For this review, take the finished solid that the model builds, in its own axes (mm). Face numbers are marked on the shaded views. Round coordinates to 2 decimals unless told otherwise and drop trailing zeros. Loops run counter-clockwise (first coordinate to the right, second up) from the corner with the lowest first, then second, coordinate; pieces in that order, holes last.
1) Mouldability with a two-part tool opening along X and no side actions: class the marked faces 1, 2 and 3 as pulls with the +X half, pulls with the -X half, needs draft (parallel to the pull), parting line crosses it, or undercut.
2) Insertion check: pin 1 (3 mm diameter, centred on x = 44.45, y = 780.22, fed in from -Z). The pin has a flat end and moves straight along its axis. Give the tip position at first contact, or say it passes through.
3) Take a section at A-A (z = 134.75). State the section outline as (x, y) points.
4) Take a section at B-B (x = 44). Give the number of separate pieces and of enclosed holes in the cut face, then the cut area to 3 significant figures.
5) Wall thickness on L1, parallel to Y at x = 41, z = 135; L2, parallel to Y at x = 40.25, z = 134.5; L3, parallel to Y at x = 46, z = 136: over which ranges is each line inside the solid? List them lowest first.
6) Take a section at C-C (z = 131.25). State the section outline as (x, y) points.
```python
from build123d import *

# Parameters (mm, degrees)
SKETCH1_W           = 9.525
SKETCH1_H           = 50.8
SKETCH1_R           = 3.175
BOSS_EXTRUDE1_DEPTH = 12.7
CUT_EXTRUDE1_REACH  = 791.849
SKETCH2_R           = 2.6035


with BuildPart() as part:
    # Sketch1 → Boss-Extrude1 (new body)
    with BuildSketch(Plane(origin=(38.1, 0, 0), x_dir=(0, 0, -1), z_dir=(1, 0, 0))):
        with Locations((-134.9375, 762.756140976)):
            Rectangle(SKETCH1_W, SKETCH1_H)
        with Locations((-134.9375, 769.106140976)):
            Circle(SKETCH1_R, mode=Mode.SUBTRACT)
        with Locations(Location((-134.9375, 756.406140976, 0), (0, 0, 180))):
            Circle(SKETCH1_R, mode=Mode.SUBTRACT)
    extrude(amount=BOSS_EXTRUDE1_DEPTH)

    # Sketch2 → Cut-Extrude1 (cut, up to next)
    with BuildSketch(Plane(origin=(0, 0, 130.175), x_dir=(-1, 0, 0), z_dir=(0, 0, -1)), mode=Mode.PRIVATE) as cut_extrude1_sk1:
        with Locations(Location((-44.45, 780.218640976, 0), (0, 0, 90))):
            Circle(SKETCH2_R)
    cut_extrude1_tool1 = extrude(cut_extrude1_sk1.sketch, amount=-CUT_EXTRUDE1_REACH, mode=Mode.PRIVATE) & part.part
    # Sketch2 → Cut-Extrude1 (cut, up to next)
    with BuildSketch(Plane(origin=(0, 0, 130.175), x_dir=(-1, 0, 0), z_dir=(0, 0, -1)), mode=Mode.PRIVATE) as cut_extrude1_sk2:
        with Locations(Location((-44.45, 745.293640976, 0), (0, 0, 90))):
            Circle(SKETCH2_R)
    cut_extrude1_tool2 = extrude(cut_extrude1_sk2.sketch, amount=-CUT_EXTRUDE1_REACH, mode=Mode.PRIVATE) & part.part
    add(cut_extrude1_tool1.solids().sort_by_distance((44.45, 780.218641, 130.175))[0], mode=Mode.SUBTRACT)
    add(cut_extrude1_tool2.solids().sort_by_distance((44.45, 745.293641, 130.175))[0], mode=Mode.SUBTRACT)


solid = part.part
```
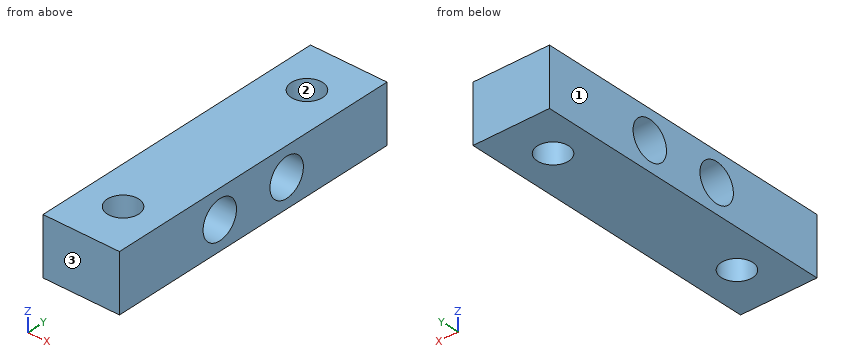
Response:
1. face 1: pulls with the -X half
1. face 2: undercut
1. face 3: needs draft
2. pin 1: passes through
3. outline: (38.1, 737.36) - (50.8, 737.36) - (50.8, 753.24) - (38.1, 753.24) - close; (38.1, 759.58) - (50.8, 759.58) - (50.8, 765.94) - (38.1, 765.94) - close; (38.1, 772.28) - (50.8, 772.28) - (50.8, 788.16) - (38.1, 788.16) - close; hole circle Ø5.21 at (44.45, 745.29); hole circle Ø5.21 at (44.45, 780.22)
4. separate pieces: 3
4. enclosed holes: 2
4. area: 323 mm2
5. L1: y = 737.36 to 753.23, 759.58 to 765.93, 772.28 to 788.16
5. L2: y = 737.36 to 753.26, 759.55 to 765.96, 772.25 to 788.16
5. L3: y = 737.36 to 743.2, 747.39 to 753.41, 759.4 to 766.11, 772.1 to 778.13, 782.31 to 788.16
6. outline: (38.1, 737.36) - (50.8, 737.36) - (50.8, 788.16) - (38.1, 788.16) - close; hole circle Ø5.21 at (44.45, 745.29); hole circle Ø5.21 at (44.45, 780.22)
